```python
from build123d import *

# Parameters (mm, degrees)
MODEL_R                  = 8.35
RESSALTO_EXTRUS_O2_DEPTH = 4
ESBO_O5_W                = 2
ESBO_O5_H                = 24
RESSALTO_EXTRUS_O3_DEPTH = 20
ESBO_O6_OUTSIDE_W        = 30.002
ESBO_O6_OUTSIDE_H        = 34.002
ESBO_O6_OUTSIDE_R        = 13
CORTE_EXTRUS_O1_DEPTH    = 26
CORTE_EXTRUS_O2_DEPTH    = 26
RESSALTO_EXTRUS_O4_DEPTH = 4
CORTE_EXTRUS_O3_DEPTH    = 20.5000001


with BuildPart() as part:
    # Model → Ressalto-extrusão2 (new body)
    with BuildSketch(Plane.XY):
        Polygon((0, 44.200000002), (0, 59.200000002), (-5.55, 59.200000002), (-5.55, 63.700000002), (-23, 63.700000002), (-23, 39.700000002), (-5.55, 39.700000002), (-5.55, 44.200000002), align=None)
        with Locations((-13.5, 51.700000002)):
            Circle(MODEL_R, mode=Mode.SUBTRACT)
    extrude(amount=RESSALTO_EXTRUS_O2_DEPTH)

    # Esboço5 → Ressalto-extrusão3 (add)
    with BuildSketch(Plane(origin=(0, 0, 0), x_dir=(-1, 0, 0), z_dir=(0, 0, -1))):
        with Locations((24, 51.700000002)):
            Rectangle(ESBO_O5_W, ESBO_O5_H)
    extrude(amount=-RESSALTO_EXTRUS_O3_DEPTH)

    # Esboço6 outside → Corte-extrusão1 (cut, through all)
    with BuildSketch(Plane.ZY.offset(25)):
        with Locations((10, 51.7)):
            Rectangle(ESBO_O6_OUTSIDE_W, ESBO_O6_OUTSIDE_H)
        with Locations((10, 51.700000002)):
            Circle(ESBO_O6_OUTSIDE_R, mode=Mode.SUBTRACT)
    extrude(amount=-CORTE_EXTRUS_O1_DEPTH, mode=Mode.SUBTRACT)

    # Esboço8 → Corte-extrusão2 (cut, through all)
    with BuildSketch(Plane.ZY.offset(25)):
        Polygon((7.885, 51.700000002), (10, 49.585000002), (12.115, 51.700000002), (10, 53.815000002), align=None)
    extrude(amount=-CORTE_EXTRUS_O2_DEPTH, mode=Mode.SUBTRACT)

    # Espelhar1: part across plane


with BuildPart() as part_1:
    add(part.part)
    add(part.part.mirror(Plane(origin=(0, 44.200000002, 4), x_dir=(0, 0, 1), z_dir=(-1, 0, 0))))

    # Esboço9 → Ressalto-extrusão4 (add)
    with BuildSketch(Plane.XY.offset(4)):
        Polygon((0, 59.200000002), (4, 59.200000002), (4, 44.200000002), (-4, 44.200000002), (-4, 59.200000002), align=None)
    extrude(amount=RESSALTO_EXTRUS_O4_DEPTH)

    # Esboço10 → Corte-extrusão3 (cut, through all)
    with BuildSketch(Plane(origin=(0, 59.200000002, 0), x_dir=(1, 0, 0), z_dir=(0, 1, 0))):
        Polygon((0, -1.885), (-2.115, -4), (0, -6.115), (2.115, -4), align=None)
    extrude(amount=-CORTE_EXTRUS_O3_DEPTH, mode=Mode.SUBTRACT)


solid = part_1.part
```
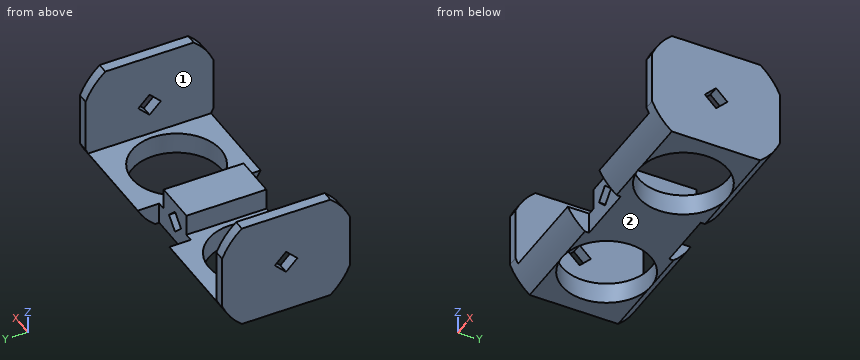
Work out the finished part from the listing and answer in its coordinate system (mm). Face numbers are marked on the shaded views. A direction names the side the tool comes from. Coordinates: 2 decimals unless noted, no trailing zeros. Loops run counter-clockwise (first coordinate to the right, second up) from the corner with the lowest first, then second, coordinate; pieces in that order, holes last. Notation, with made-up numbers: (12, 10.25) -> (59, 10.25) arc R30 ccw to (59, 33.25) -> close; hole circle Ø9 at (31, -4.5). An arc over 180 degrees is marked (long way). Answer as CSV lines item,"result".
Q1. Each of these flat-tipped pins is pushed along its axis until it touches: pin 1 (6 mm diameter, centred on x = -10, y = 58.5, fed in from +Z); pin 2 (6.5 mm diameter, centred on x = 0.5, z = 4, fed in from +Y); pin 3 (9 mm diameter, centred on x = 0, y = 53, fed in from +Z). Where does it stop, or does it pass through?
Findings:
pin 1,"stops at z = 4"
pin 2,"stops at y = 59.2"
pin 3,"stops at z = 8"
Q2. The part is cut by section D-D on z = 3.5. Write down the section's boundary in (x, y) (3 decimals).
Findings:
outline,"(-25, 40.442) -> (-5.55, 40.442) -> (-5.55, 44.2) -> (-1.615, 44.2) -> (-1.615, 59.2) -> (-5.55, 59.2) -> (-5.55, 62.958) -> (-25, 62.958) -> close; (1.615, 44.2) -> (5.55, 44.2) -> (5.55, 40.442) -> (25, 40.442) -> (25, 62.958) -> (5.55, 62.958) -> (5.55, 59.2) -> (1.615, 59.2) -> close; hole circle Ø16.7 at (-13.5, 51.7); hole circle Ø16.7 at (13.5, 51.7)"
Q3. The part is cut by section A-A on z = 13.25. Write down the section's boundary in (x, y).
Findings:
outline,"(-25, 39.7) -> (-23, 39.7) -> (-23, 63.7) -> (-25, 63.7) -> close; (23, 39.7) -> (25, 39.7) -> (25, 63.7) -> (23, 63.7) -> close"
Q4. A tool of negligible diameter and unlimited length cuts with its end or side. For the marked faces 1 and 2, from which of +Z, -Z, +X, -X, +Y, -Y can it reach the whole face along a straight path? Write none if from no direction.
Findings:
face 1,"+Z, +Y, -Y"
face 2,"-Z, +X, -X, +Y, -Y"
Q5. The part is cut by section C-C on x = -11. Write down the section's boundary in (y, z), and give its area (3 significant figures).
Findings:
outline,"(40.17, 4) arc R13 ccw to (43.39, 0) -> (43.73, 0) -> (43.73, 4) -> close; (59.67, 0) -> (60.01, 0) arc R13 ccw to (63.23, 4) -> (59.67, 4) -> close"
area,"17.4 mm²"
Q6. The part is cut by section B-B on y = 46. Write down the section's boundary in (x, z) (3 decimals).
Findings:
outline,"(-25, 0) -> (-19.602, 0) -> (-19.602, 4) -> (-23, 4) -> (-23, 20) -> (-25, 20) -> close; (-7.398, 0) -> (7.398, 0) -> (7.398, 4) -> (4, 4) -> (4, 8) -> (-4, 8) -> (-4, 4) -> (-7.398, 4) -> close; (19.602, 0) -> (25, 0) -> (25, 20) -> (23, 20) -> (23, 4) -> (19.602, 4) -> close; hole (-2.115, 4) -> (0, 1.885) -> (2.115, 4) -> (0, 6.115) -> close"
Q7. Find the intervals of material crossed by probe 1 along X at (y, z) = (45, 6.25); probe 2 along X at (y, z) = (55, 5.25) (3 decimals); probe 3 along X at (y, z) = (53.5, 5) (3 decimals), in increasing order.
Findings:
probe 1,"x = -25 to -23, -4 to 4, 23 to 25"
probe 2,"x = -25 to -23, -4 to -0.865, 0.865 to 4, 23 to 25"
probe 3,"x = -25 to -23, -4 to -1.115, 1.115 to 4, 23 to 25"
